Build history of the part. All positions in model axes, mm. Round coordinates to 2 decimals unless told otherwise and drop trailing zeros. Order: outer loops, then holes, each group sorted by start corner. A loop starts at its lowest first (then second) coordinate and runs counter-clockwise, first axis right, second up. Notation, with made-up numbers: (-19.75, 89.25) -> (27.25, 89.25) arc R8 cw to (27.25, 97.25) -> close; hole circle Ø11 at (37, -20). An arc over 180 degrees is marked (long way). Write item = value, one per line.
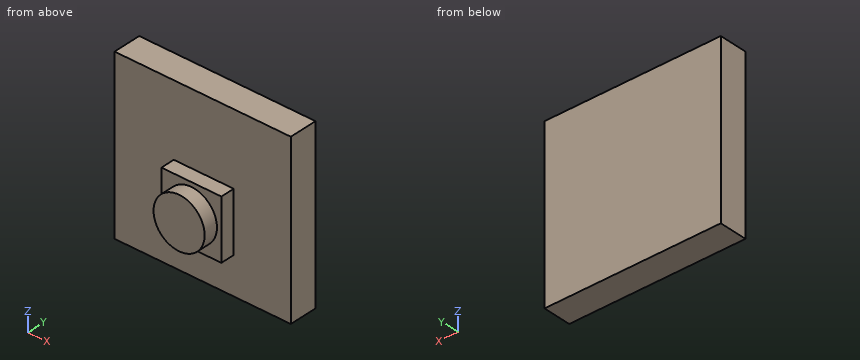
from build123d import *

# Parameters (mm, degrees)
F0_W     = 25
F0_H     = 24
F1_DEPTH = 2
F2_W     = 8.5
F2_H     = 8.5
F3_DEPTH = 2
F4_R     = 3.625
F5_DEPTH = 2


with BuildPart() as f1:
    # F0 (on Front) → F1 (new body, symmetric)
    with BuildSketch(Plane.XZ):
        Rectangle(F0_W, F0_H)
    extrude(amount=F1_DEPTH, both=True)

    # F2 (on face) → F3 (join)
    with BuildSketch(Plane.XZ.offset(2)):
        with Locations((0.15, -2.45)):
            Rectangle(F2_W, F2_H)
    extrude(amount=F3_DEPTH)

    # F4 (on face) → F5 (join)
    with BuildSketch(Plane.XZ.offset(4)):
        with Locations((0.15, -2.45)):
            Circle(F4_R)
    extrude(amount=F5_DEPTH)


solid = f1.part
Q1. Cut at B-B, the plane x = 0.15. List the corners of the cut face in (y, z) (3 decimals).
Check values:
outline = (-6, -6.075) -> (-4, -6.075) -> (-4, -6.7) -> (-2, -6.7) -> (-2, -12) -> (2, -12) -> (2, 12) -> (-2, 12) -> (-2, 1.8) -> (-4, 1.8) -> (-4, 1.175) -> (-6, 1.175) -> close
Q2. Cut at D-D, the plane x = -8. List the corners of the cut face in (y, z), and give its area (3 significant figures).
Check values:
outline = (-2, -12) -> (2, -12) -> (2, 12) -> (-2, 12) -> close
area = 96.0 mm²
Q3. Cut at C-C, the plane y = -4.5. List the corners of the cut face in (x, z) (3 decimals), and give its area (3 significant figures).
Check values:
outline = circle Ø7.25 at (0.15, -2.45)
area = 41.3 mm²
Q4. Cut at A-A, the plane z = -2.45. List the corners of the cut face in (x, y) (3 decimals).
Check values:
outline = (-12.5, -2) -> (-4.1, -2) -> (-4.1, -4) -> (-3.475, -4) -> (-3.475, -6) -> (3.775, -6) -> (3.775, -4) -> (4.4, -4) -> (4.4, -2) -> (12.5, -2) -> (12.5, 2) -> (-12.5, 2) -> close
Q5. Probe probe 1 along Y at (x, z) = (9.25, 3.5); probe 2 along Y at (x, z) = (4, -2.75); probe 3 along Z at (x, y) = (3.25, -3.5). List the from-to ranges inside material, lowest first.
Check values:
probe_1 = -2 to 2
probe_2 = -4 to 2
probe_3 = -6.7 to 1.8
Q6. Flat gauge pins, fed straight in: pin 1 (1 mm diameter, centred on x = -1, y = -3.5, fed in from +Z); pin 2 (7 mm diameter, centred on x = 1.5, z = 6, fed in from -Y); pin 3 (0.6 mm diameter, centred on y = -3, z = -4, fed in from +X). Where does each tip first touch, or does it go through?
Check values:
pin_1 = 1.8
pin_2 = -2
pin_3 = 4.4
